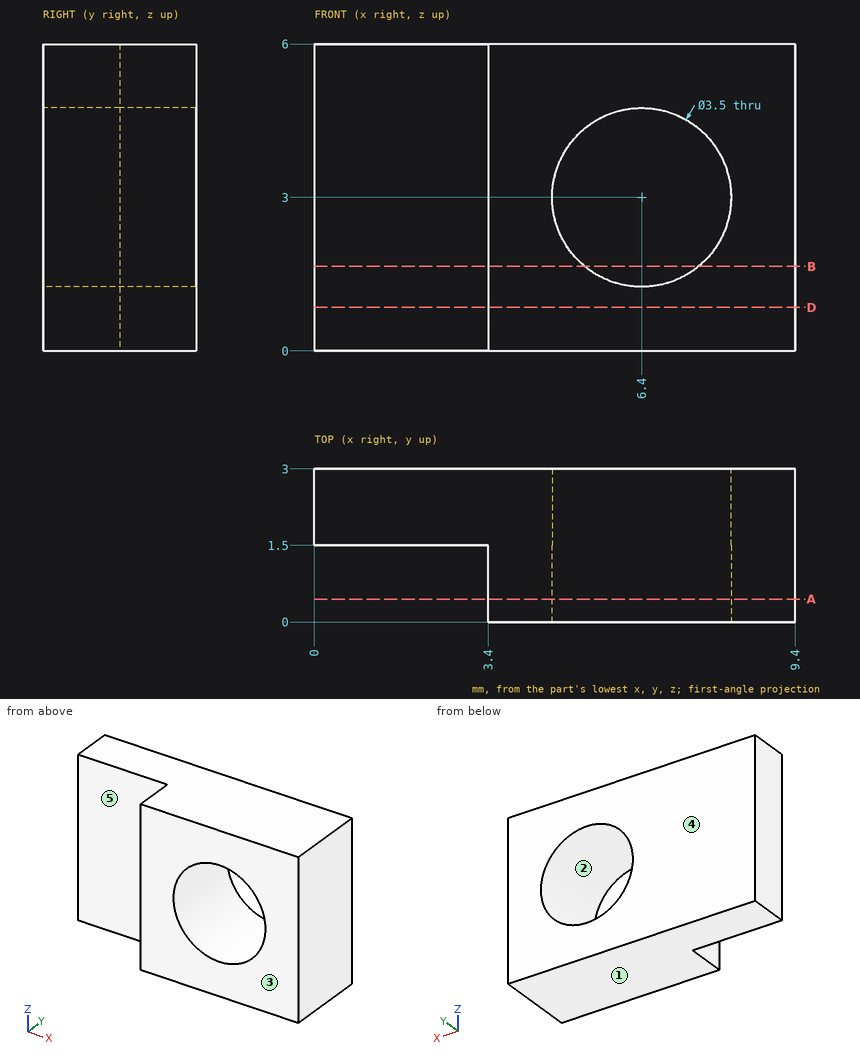
Part print with two shaded views. Sizes in mm from the minimum x, y, z corner. A direction names the side the tool comes from. Coordinates: 2 decimals unless noted, no trailing zeros. Write each loop counter-clockwise with the first axis right and the second up, starting at its lowest first coordinate (ties: lowest second). Pieces come first, ordered by that corner, then holes. Notation, with made-up numbers: (-36, 44.5) - (17, 44.5) arc R23 ccw to (17, 83.5) - close; hole circle Ø4 at (-3.5, 59.25). An arc over 180 degrees is marked (long way). Put each result on its own line as item: value.
1. Flat gauge pins, fed straight in: pin 1 Ø1.7 at (x, z) = (2.5, 3) entering from -Y; pin 2 Ø0.8 at (y, z) = (0.5, 2.5) entering from -X. Where does each tip first touch, or does it go through?
Final values:
pin 1: stops at y = 1.5
pin 2: stops at x = 3.4
2. Band-saw the part on B-B (z = 1.65). Write the cut outline in (x, y).
Final values:
outline: (0, 1.5) - (3.4, 1.5) - (3.4, 0) - (5.29, 0) - (5.29, 3) - (0, 3) - close; (7.51, 0) - (9.4, 0) - (9.4, 3) - (7.51, 3) - close
3. 3-axis set-ups, long thin cutter, end or side, ignore diameter. For the marked faces 4 and 5: which of +Z, -Z, +X, -X, +Y, -Y reach the whole face in a straight line?
Final values:
face 4: +Z, -Z, +X, -X, +Y
face 5: +Z, -Z, -X, -Y
4. Two-plate mould, pull along Z, no slides. Class the marked faces 1, 2 and 3: +Z half, -Z half, draft (parallel to the pull), parting line (faces both ways), or undercut.
Final values:
face 1: -Z half
face 2: undercut
face 3: draft
5. Band-saw the part on A-A (y = 0.45). Write the cut outline in (x, z), then the cut area to 3 significant figures.
Final values:
outline: (3.4, 0) - (9.4, 0) - (9.4, 6) - (3.4, 6) - close; hole circle Ø3.5 at (6.4, 3)
area: 26.4 mm²
6. Band-saw the part on D-D (z = 0.85). Write the cut outline in (x, y), then the cut area to 3 significant figures.
Final values:
outline: (0, 1.5) - (3.4, 1.5) - (3.4, 0) - (9.4, 0) - (9.4, 3) - (0, 3) - close
area: 23.1 mm²
7. Probe line 1 along X through (y, z) = (2, 3); line 2 along Z through (x, y) = (6.4, 1.05); line 3 along X through (y, z) = (0.95, 3). List the from-to ranges inside material, lowest first. Write a range as [from, to].
Final values:
line 1: x = [0, 4.65], [8.15, 9.4]
line 2: z = [0, 1.25], [4.75, 6]
line 3: x = [3.4, 4.65], [8.15, 9.4]
